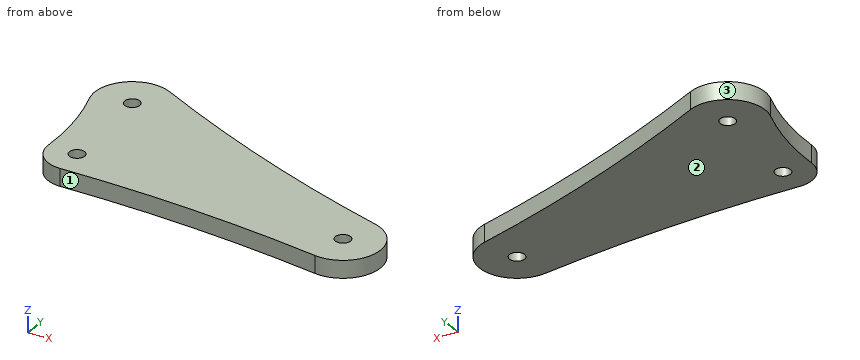
from build123d import *

# Parameters (mm, degrees)
SKETCH1_R           = 1.525
BOSS_EXTRUDE1_DEPTH = 3.5


with BuildPart() as part:
    # Sketch1 → Boss-Extrude1 (new body)
    with BuildSketch(Plane.XY):
        with BuildLine():
            ThreePointArc((-5.798114447, 0.147881218), (-4.091440025, -4.110975374), (0.175497637, -5.79734427))
            ThreePointArc((0.175497637, -5.79734427), (26.625773358, -6.107804645), (52.956740344, -8.636371224))
            ThreePointArc((52.956740344, -8.636371224), (61.328682163, -2.737878642), (56.01066855, 6.014284277))
            ThreePointArc((56.01066855, 6.014284277), (28.510221344, 15.105334328), (1.961063899, 26.683936423))
            ThreePointArc((1.961063899, 26.683936423), (-6.300180669, 25.588718748), (-8.449807785, 17.537211633))
            ThreePointArc((-8.449807785, 17.537211633), (-6.353241495, 8.96007321), (-5.798114447, 0.147881218))
        make_face()
        with Locations((-1.35, 19.954385483)):
            Circle(SKETCH1_R, mode=Mode.SUBTRACT)
        Circle(SKETCH1_R, mode=Mode.SUBTRACT)
        with Locations((53.9865, -1.207401238)):
            Circle(SKETCH1_R, mode=Mode.SUBTRACT)
    extrude(amount=BOSS_EXTRUDE1_DEPTH)


solid = part.part
Input: part model. Units: mm. Frame: model coordinates. Face numbers are marked on the shaded views. Round coordinates to 2 decimals unless told otherwise and drop trailing zeros. Order: outer loops, then holes, each group sorted by start corner. A loop starts at its lowest first (then second) coordinate and runs counter-clockwise, first axis right, second up. Notation, with made-up numbers: (-3, 7) - (3, 7) arc R22 cw to (3, 28) - close; hole circle Ø4 at (83, 8). An arc over 180 degrees is marked (long way). Use a Markdown table: item, result.
1. First-contact query: pin 1 (4 mm diameter, centred on x = 53.99, y = -1.21, fed in from +Z); pin 2 (2 mm diameter, centred on x = 35, z = 0.5, fed in from +Y); pin 3 (1 mm diameter, centred on y = 12.5, z = 1.5, fed in from -X); pin 4 (2 mm diameter, centred on x = 8, z = 1.5, fed in from -Y). Flat tips, straight axial feed; report the tip coordinate or a pass-through.
Evaluation:
| item | result |
|---|---|
| pin 1 | z = 3.5 |
| pin 2 | y = 13.06 |
| pin 3 | x = -7.14 |
| pin 4 | y = -5.66 |
2. Section A-A on z = 2.4. State how many separate pieces and enclosed holes the cut face has, then the cut area to 3 significant figures.
Evaluation:
| item | result |
|---|---|
| separate pieces | 1 |
| enclosed holes | 3 |
| area | 1,510 mm^2 |
3. Material intervals for probe 1 along Y at (x, z) = (0, 1.45) (3 decimals); probe 2 along X at (y, z) = (20, 2.8); probe 3 along X at (y, z) = (1, 0.7), sorted ascending.
Evaluation:
| item | result |
|---|---|
| probe 1 | -5.8 to -1.525, 1.525 to 19.245, 20.664 to 27.332 |
| probe 2 | -8.85 to -2.87, 0.17 to 16.46 |
| probe 3 | -5.78 to -1.15, 1.15 to 61.15 |
4. Section C-C on x = 44. Return the cut outline in (y, z).
Evaluation:
| item | result |
|---|---|
| outline | (-7.53, 0) - (9.64, 0) - (9.64, 3.5) - (-7.53, 3.5) - close |
5. Section B-B on x = 54. Return the cut outline in (y, z).
Evaluation:
| item | result |
|---|---|
| outline | (-8.71, 0) - (-2.73, 0) - (-2.73, 3.5) - (-8.71, 3.5) - close; (0.32, 0) - (6.59, 0) - (6.59, 3.5) - (0.32, 3.5) - close |
6. Mould query, pull axis X, two halves, no side actions, for the marked faces 1, 2 and 3. Classes: +X half, -X half, draft (parallel to the pull), parting line (faces both ways), or undercut.
Evaluation:
| item | result |
|---|---|
| face 1 | undercut |
| face 2 | draft |
| face 3 | parting line |
7. Section D-D on y = 12. Return the cut outline in (x, z), then the cut area to 3 significant figures.
Evaluation:
| item | result |
|---|---|
| outline | (-6.91, 0) - (36.99, 0) - (36.99, 3.5) - (-6.91, 3.5) - close |
| area | 154 mm^2 |
